Geometry: final body of the model. Coordinates: model frame, mm. Face numbers are marked on the shaded views. Round coordinates to 2 decimals unless told otherwise and drop trailing zeros. Order: outer loops, then holes, each group sorted by start corner. A loop starts at its lowest first (then second) coordinate and runs counter-clockwise, first axis right, second up. Notation, with made-up numbers: (20, -29.5) -> (60, -29.5) arc R13 cw to (60, -10.5) -> close; hole circle Ø8 at (-34, -39). An arc over 180 degrees is marked (long way). Put each result on its own line as item: value.
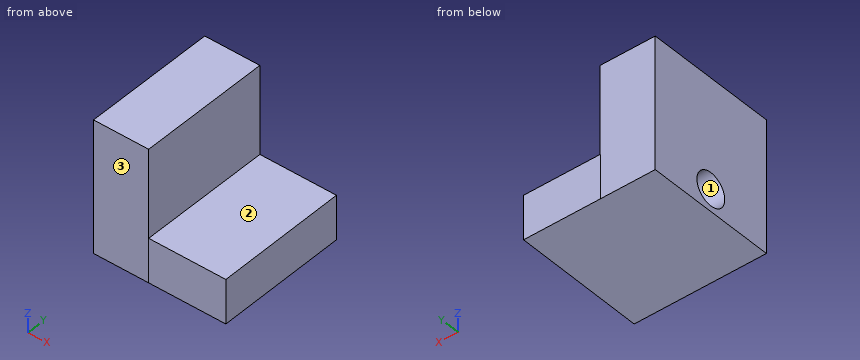
```python
from build123d import *

# Parameters (mm, degrees)
F0_W     = 25
F0_H     = 60
F1_DEPTH = 60
F3_DEPTH = 20
F5_D     = 15
F5_DEPTH = 20
F5_TIP   = 4.5064546427


with BuildPart() as f1:
    # F0 (on Top) → F1 (new body)
    with BuildSketch(Plane.XY):
        with Locations((-17.5, 0)):
            Rectangle(F0_W, F0_H)
    extrude(amount=F1_DEPTH)

    # F2 (on Top) → F3 (join)
    with BuildSketch(Plane.XY):
        Polygon((29.7366095148, 30.0084589422), (-5.2633904852, 30.0084589422), (-4.995259922, -29.9915410578), (30.004740078, -29.9915410578), align=None)
    extrude(amount=F3_DEPTH)

    # F5
    with Locations(Plane(origin=(-30, 0, 0), x_dir=(0, -1, 0), z_dir=(-1, 0, 0))):
        with Locations((0, 10)):
            Hole(F5_D / 2, depth=F5_DEPTH)
            with Locations((0, 0, -(F5_DEPTH + F5_TIP / 2))):  # 118° drill point
                Cone(0, F5_D / 2, F5_TIP, mode=Mode.SUBTRACT)


solid = f1.part
```
1. Cut plane C-C on y = -17.5. Return loops of the section in (x, z), and give its area (3 significant figures).
Ans:
outline: (-30, 0) -> (29.95, 0) -> (29.95, 20) -> (-5, 20) -> (-5, 60) -> (-30, 60) -> close
area: 2,200 mm²
2. Material intervals for probe 1 along Y at (x, z) = (-19, 10); probe 2 along Z at (x, y) = (-19.25, 0); probe 3 along Z at (x, y) = (9.5, 21), sorted ascending.
Ans:
probe 1: -30 to -7.5, 7.5 to 30
probe 2: 0 to 2.5, 17.5 to 60
probe 3: 0 to 20
3. Contact query for flat-ended pins moving along their axis: P1, Ø12.5, axis at x = -13, z = 41, coming from the +Y side; P2, Ø22, axis at x = 20, z = 14, coming from the -Y side; P3, Ø1.5, axis at x = 20, y = 7.5, coming from the +Z side; P4, Ø6, axis at x = -23, y = -10, coming from the -Z side. Output: stop coordinate, or through.
Ans:
P1: y = 30
P2: y = -29.99
P3: z = 20
P4: z = 0
4. Cut plane B-B on z = 29.5. Return loops of the section in (x, y), and give its area (3 significant figures).
Ans:
outline: (-30, -30) -> (-5, -30) -> (-5, 30) -> (-30, 30) -> close
area: 1,500 mm²
5. Cut plane A-A on x = -18. Return loops of the section in (y, z).
Ans:
outline: (-30, 0) -> (30, 0) -> (30, 60) -> (-30, 60) -> close; hole circle Ø15 at (0, 10)
6. Cut plane D-D on x = 20. Return loops of the section in (y, z).
Ans:
outline: (-29.99, 0) -> (30.01, 0) -> (30.01, 20) -> (-29.99, 20) -> close
7. Draft query along Y for the marked faces 1, 2 and 3. Return one class per face: +Y half, -Y half, draft (parallel to the pull), parting line (faces both ways), or undercut.
Ans:
face 1: undercut
face 2: draft
face 3: -Y half
